```python
from build123d import *

# Parameters (mm, degrees)
BOSS_EXTRUDE1_DEPTH        = 1.5
BOSS_EXTRUDE1_DEPTH_BACK   = 1.5
BOSS_EXTRUDE1_2_DEPTH      = 1.5
BOSS_EXTRUDE1_2_DEPTH_BACK = 1.5
BOSS_EXTRUDE1_3_DEPTH      = 1.5
BOSS_EXTRUDE1_3_DEPTH_BACK = 1.5
BOSS_EXTRUDE1_4_DEPTH      = 1.5
BOSS_EXTRUDE1_4_DEPTH_BACK = 1.5
BOSS_EXTRUDE2_DEPTH        = 1.5


with BuildPart() as part:
    # Sketch1 → Boss-Extrude1 (new, two sides: drawn at the far end of the back side and taken through both)
    with BuildSketch(Plane(origin=(0, 0, 0), x_dir=(1, 0, 0), z_dir=(0, 1, 0)).offset(-BOSS_EXTRUDE1_DEPTH_BACK)):
        with BuildLine():
            Line((2.279435677, 3.764359918), (6.75753788, 8.24246212))
            ThreePointArc((6.75753788, 8.24246212), (0, 5.613736217), (-6.75753788, 8.24246212))
            Line((-6.75753788, 8.24246212), (-2.279435677, 3.764359918))
            ThreePointArc((-2.279435677, 3.764359918), (0, 2.935880264), (2.279435677, 3.764359918))
        make_face()
    extrude(amount=BOSS_EXTRUDE1_DEPTH + BOSS_EXTRUDE1_DEPTH_BACK)



with BuildPart() as body_2:
    # Sketch1 → Boss-Extrude1 2 (new, two sides: drawn at the far end of the back side and taken through both)
    with BuildSketch(Plane(origin=(0, 0, 0), x_dir=(1, 0, 0), z_dir=(0, 1, 0)).offset(-BOSS_EXTRUDE1_2_DEPTH_BACK)):
        with BuildLine():
            Line((-8.24246212, 6.75753788), (-3.764359918, 2.279435677))
            ThreePointArc((-3.764359918, 2.279435677), (-2.935880264, 0), (-3.764359918, -2.279435677))
            Line((-3.764359918, -2.279435677), (-8.24246212, -6.75753788))
            ThreePointArc((-8.24246212, -6.75753788), (-5.613736217, 0), (-8.24246212, 6.75753788))
        make_face()
    extrude(amount=BOSS_EXTRUDE1_2_DEPTH + BOSS_EXTRUDE1_2_DEPTH_BACK)


with BuildPart() as body_3:
    # Sketch1 → Boss-Extrude1 3 (new, two sides: drawn at the far end of the back side and taken through both)
    with BuildSketch(Plane(origin=(0, 0, 0), x_dir=(1, 0, 0), z_dir=(0, 1, 0)).offset(-BOSS_EXTRUDE1_3_DEPTH_BACK)):
        with BuildLine():
            Line((-6.75753788, -8.24246212), (-2.279435677, -3.764359918))
            ThreePointArc((-2.279435677, -3.764359918), (0, -2.935880264), (2.279435677, -3.764359918))
            Line((2.279435677, -3.764359918), (6.75753788, -8.24246212))
            ThreePointArc((6.75753788, -8.24246212), (0, -5.613736217), (-6.75753788, -8.24246212))
        make_face()
    extrude(amount=BOSS_EXTRUDE1_3_DEPTH + BOSS_EXTRUDE1_3_DEPTH_BACK)


with BuildPart() as body_4:
    # Sketch1 → Boss-Extrude1 4 (new, two sides: drawn at the far end of the back side and taken through both)
    with BuildSketch(Plane(origin=(0, 0, 0), x_dir=(1, 0, 0), z_dir=(0, 1, 0)).offset(-BOSS_EXTRUDE1_4_DEPTH_BACK)):
        with BuildLine():
            Line((3.764359918, -2.279435677), (8.24246212, -6.75753788))
            ThreePointArc((8.24246212, -6.75753788), (5.613736217, 0), (8.24246212, 6.75753788))
            Line((8.24246212, 6.75753788), (3.764359918, 2.279435677))
            ThreePointArc((3.764359918, 2.279435677), (2.935880264, 0), (3.764359918, -2.279435677))
        make_face()
    extrude(amount=BOSS_EXTRUDE1_4_DEPTH + BOSS_EXTRUDE1_4_DEPTH_BACK)


with BuildPart() as part_1:
    add(part.part)

    add(body_2.part)  # Boss-Extrude2 merges body 2

    add(body_3.part)  # Boss-Extrude2 merges body 3

    add(body_4.part)  # Boss-Extrude2 merges body 4
    # Sketch1_4 → Boss-Extrude2 (add)
    with BuildSketch(Plane(origin=(0, 0, 0), x_dir=(1, 0, 0), z_dir=(0, 1, 0))):
        with BuildLine():
            Line((2.279435677, 3.764359918), (6.75753788, 8.24246212))
            Line((6.75753788, 8.24246212), (8.24246212, 6.75753788))
            Line((8.24246212, 6.75753788), (3.764359918, 2.279435677))
            ThreePointArc((3.764359918, 2.279435677), (2.935880264, 0), (3.764359918, -2.279435677))
            Line((3.764359918, -2.279435677), (8.24246212, -6.75753788))
            Line((8.24246212, -6.75753788), (6.75753788, -8.24246212))
            Line((6.75753788, -8.24246212), (2.279435677, -3.764359918))
            ThreePointArc((2.279435677, -3.764359918), (0, -2.935880264), (-2.279435677, -3.764359918))
            Line((-2.279435677, -3.764359918), (-6.75753788, -8.24246212))
            Line((-6.75753788, -8.24246212), (-8.24246212, -6.75753788))
            Line((-8.24246212, -6.75753788), (-3.764359918, -2.279435677))
            ThreePointArc((-3.764359918, -2.279435677), (-2.935880264, 0), (-3.764359918, 2.279435677))
            Line((-3.764359918, 2.279435677), (-8.24246212, 6.75753788))
            Line((-8.24246212, 6.75753788), (-6.75753788, 8.24246212))
            Line((-6.75753788, 8.24246212), (-2.279435677, 3.764359918))
            ThreePointArc((-2.279435677, 3.764359918), (0, 2.935880264), (2.279435677, 3.764359918))
        make_face()
    extrude(amount=BOSS_EXTRUDE2_DEPTH)


solid = part_1.part
```
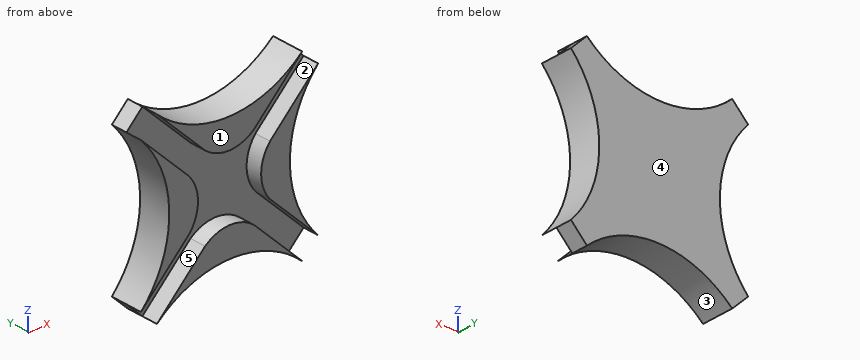
The listing builds one solid part. Answer for the finished solid, in the listing's coordinates (mm). Face numbers are marked on the shaded views. A direction names the side the tool comes from. Give positions to 0.01 mm unless a question says otherwise; leave off trailing zeros. Loops run counter-clockwise (first coordinate to the right, second up) from the corner with the lowest first, then second, coordinate; pieces in that order, holes last. Notation, with made-up numbers: (84, -25.75) - (114, -25.75) arc R9 cw to (114, -20.75) - close; hole circle Ø7 at (44.25, -38.75). An arc over 180 degrees is marked (long way). Return JSON: item names as keys, results as strings. Group by question number.
1. Given pin 1 Ø1 at (y, z) = (0, 3) entering from -X; pin 2 Ø1 at (x, y) = (-2.5, -1) entering from -Z, each flat-ended and moving along its own axis, determine where each tip first touches the part or whether it passes through.
2. Determine the mould class of the marked faces 1, 2 and 3 for opening direction Z: pulls with the +Z half, pulls with the -Z half, needs draft (parallel to the pull), parting line crosses it, or undercut.
3. Find section D-D (y = 0.45). Write down the section's boundary in (x, z), then the cut area to 3 significant figures.
4. Find section A-A (y = -1.3). Write down the section's boundary in (x, z).
5. Find section C-C (z = -6). Write down the section's boundary in (x, y).
6. Which of the six approach directions +Z, -Z, +X, -X, +Y, -Y give full straight-line access (tool end or side, diameter ignored) to the marked faces 4 and 5?
7. Straight lines are drawn through the part: line 1 (X direction, y = -1.1, z = 5); line 2 (Z direction, x = 4, y = -0.65). For each, find the intervals that lie inside material, in ascending order. Write a range as [from, to].
Verdict:
{
 "1": {"pin 1": "stops at x = -6.25", "pin 2": "stops at z = -6.07"},
 "2": {"face 1": "needs draft", "face 2": "undercut", "face 3": "pulls with the -Z half"},
 "3": {"outline": "(-8.24, -6.76) - (-6.76, -8.24) arc R10 cw to (6.76, -8.24) - (8.24, -6.76) arc R10 cw to (8.24, 6.76) - (6.76, 8.24) arc R10 cw to (-6.76, 8.24) - (-8.24, 6.76) arc R10 cw to start", "area": "170 mm^2"},
 "4": {"outline": "(-8.24, -6.76) - (-3.76, -2.28) arc R3.55 ccw to (-3.76, 2.28) - (-8.24, 6.76) arc R10 cw to start; (-6.76, -8.24) arc R10 cw to (6.76, -8.24) - (2.28, -3.76) arc R3.55 ccw to (-2.28, -3.76) - close; (-6.76, 8.24) - (-2.28, 3.76) arc R3.55 ccw to (2.28, 3.76) - (6.76, 8.24) arc R10 cw to start; (3.76, -2.28) - (8.24, -6.76) arc R10 cw to (8.24, 6.76) - (3.76, 2.28) arc R3.55 ccw to start"},
 "5": {"outline": "(-7.61, -1.5) - (-7.48, -1.5) - (-7.48, 0) - (-4.52, 0) - (-4.52, -1.5) - (-2.75, -1.5) - (-2.75, 1.5) - (-7.61, 1.5) - close; (2.75, -1.5) - (4.52, -1.5) - (4.52, 0) - (7.48, 0) - (7.48, -1.5) - (7.61, -1.5) - (7.61, 1.5) - (2.75, 1.5) - close"},
 "6": {"face 4": "+Z, -Z, +X, -X, +Y", "face 5": "-Y"},
 "7": {"line 1": "x = [-6.95, -6.48], [-3.52, 3.52], [6.48, 6.95]", "line 2": "z = [-6.45, -5.48], [-2.52, 2.52], [5.48, 6.45]"}
}
